Model file for the job. Use its own axes, mm. A direction names the side the tool comes from. Round coordinates to 2 decimals unless told otherwise and drop trailing zeros. Loops run counter-clockwise (first coordinate to the right, second up) from the corner with the lowest first, then second, coordinate; pieces in that order, holes last. Notation, with made-up numbers: M 53.5,75.5 L 68.5,75.5 A15 cw 68.5,94.5 Z; hole C 66,-4 d7. An arc over 180 degrees is marked long. Use a Markdown table: item, result. Add a question column.
Item 1: Pin check, flat tips, straight feed: P1, Ø1, axis at x = -95, z = 9, coming from the +Y side; P2, Ø1.5, axis at x = -96, y = 41.5, coming from the +Z side; P3, Ø2, axis at y = 33, z = 11.5, coming from the +X side; P4, Ø2.5, axis at x = -86, y = 40, coming from the +Z side. Stop position of each tip, or through.
Item 2: Tool access for faces 1 (the flat face through (-96.18, 33.99, 11.52)), 2 (the flat face through (-84.7, 38.7, 13)): list every direction of +Z, -Z, +X, -X, +Y, -Y with a clear straight run to the whole face (end or side of a thin tool).
Item 3: Saw through at C-C on x = -93. Write the cut outline in (y, z).
Item 4: Wall check: L1, parallel to X at y = 40, z = 9.45; L2, parallel to X at y = 40, z = 10.7; L3, parallel to Y at x = -93, z = 9.45. Give the ranges that are in metal, low to high. Write a range as from..to.
Item 5: Two-plate mould, pull along X, no slides. Class faces 3 (the flat face through (-89.82, 46.01, 11.52)), 4 (the flat face through (-93, 43, 8)), 5 (the cylindrical face through (-89.99, 49.536, 10.465)): +X half, -X half, draft (parallel to the pull), parting line (faces both ways), or undercut.
Item 6: Saw through at A-A on y = 40. Write the cut outline in (x, z).
Item 7: Saw through at B-B on z = 10.8. Write the cut outline in (x, y).
Item 8: Saw through at D-D on x = -99.5. Write the cut outline in (y, z), then the cut area to 3 significant figures.
```python
from build123d import *

# Parameters (mm, degrees)
SKETCH042_R             = 10
PAD013_DEPTH            = 5
POCKET026_DEPTH         = 3
SKETCH044_R             = 2.75
POCKET027_DEPTH         = 5.001
SKETCH045_R             = 1.6
POCKET028_DEPTH         = 5.001
BODY008_PLACEMENT_ANGLE = 135


with BuildPart() as part:
    # Sketch042 → Pad013 (new body)
    with BuildSketch(Plane.XY):
        Circle(SKETCH042_R)
    extrude(amount=PAD013_DEPTH)

    # Sketch043 (on Face3 of Pad013) → Pocket026 (cut)
    with BuildSketch(Plane.XY.offset(5)):
        with BuildLine():
            Line((-2, 10), (2, 10))
            Line((2, 10), (2, 3.3))
            ThreePointArc((2, 3.3), (2.380761, 2.380761), (3.3, 2))
            Line((3.3, 2), (10, 2))
            Line((10, 2), (10, -2))
            Line((10, -2), (3.3, -2))
            ThreePointArc((3.3, -2), (2.380761, -2.380761), (2, -3.3))
            Line((2, -3.3), (2, -10))
            Line((2, -10), (-2, -10))
            Line((-2, -10), (-2, -3.3))
            ThreePointArc((-2, -3.3), (-2.380761, -2.380761), (-3.3, -2))
            Line((-3.3, -2), (-10, -2))
            Line((-10, -2), (-10, 2))
            Line((-10, 2), (-3.3, 2))
            ThreePointArc((-3.3, 2), (-2.380761, 2.380761), (-2, 3.3))
            Line((-2, 3.3), (-2, 10))
        make_face()
    extrude(amount=-POCKET026_DEPTH, mode=Mode.SUBTRACT)

    # Sketch044 (on Face2 of Pocket026) → Pocket027 (cut, through all)
    with BuildSketch(Plane(origin=(0, 0, 0), x_dir=(1, 0, 0), z_dir=(0, 0, -1))):
        Circle(SKETCH044_R)
    extrude(amount=-POCKET027_DEPTH, mode=Mode.SUBTRACT)

    # Sketch045 (on Face8 of Pocket027) → Pocket028 (cut, through all)
    with BuildSketch(Plane.XY.offset(5)):
        with Locations((4.949747, 4.949747)):
            Circle(SKETCH045_R)
        with Locations((-4.949747, -4.949747)):
            Circle(SKETCH045_R)
    extrude(amount=-POCKET028_DEPTH, mode=Mode.SUBTRACT)


with BuildPart() as part_1:
    # Body008 placement: moved
    add(part.part.moved(Location((-93, 40, 8))).rotate(Axis((-93, 40, 8), (0, 0, 1)), BODY008_PLACEMENT_ANGLE))


solid = part_1.part
```
Entries:
| question | item | result |
|---|---|---|
| 1 | P1 | y = 49.89 |
| 1 | P2 | z = 10 |
| 1 | P3 | x = -87.83 |
| 1 | P4 | through |
| 2 | face 1 | +Z |
| 2 | face 2 | +Z, +X, -X, +Y, -Y |
| 3 | outline | M 30,8 L 37.25,8 L 37.25,10 L 36.63,10 L 36.63,13 L 30,13 Z; M 42.75,8 L 50,8 L 50,13 L 43.37,13 L 43.37,10 L 42.75,10 Z |
| 4 | L1 | -103..-101.6, -98.4..-95.75, -90.25..-87.6, -84.4..-83 |
| 4 | L2 | -103..-101.6, -98.4..-96.37, -89.63..-87.6, -84.4..-83 |
| 4 | L3 | 30..37.25, 42.75..50 |
| 5 | face 3 | undercut |
| 5 | face 4 | draft |
| 5 | face 5 | parting line |
| 6 | outline | M -103,8 L -101.6,8 L -101.6,13 L -103,13 Z; M -98.4,8 L -95.75,8 L -95.75,10 L -96.37,10 L -96.37,13 L -98.4,13 Z; M -90.25,8 L -87.6,8 L -87.6,13 L -89.63,13 L -89.63,10 L -90.25,10 Z; M -84.4,8 L -83,8 L -83,13 L -84.4,13 Z |
| 7 | outline | M -101.34,34.49 L -96.75,39.08 A1.3 ccw -96.75,40.92 L -101.34,45.51 A10 ccw Z; M -98.51,31.66 A10 ccw -87.49,31.66 L -92.08,36.25 A1.3 ccw -93.92,36.25 Z; M -98.51,48.34 L -93.92,43.75 A1.3 ccw -92.08,43.75 L -87.49,48.34 A10 ccw Z; M -89.25,39.08 L -84.66,34.49 A10 ccw -84.66,45.51 L -89.25,40.92 A1.3 ccw Z; hole C -100,40 d3.2; hole C -86,40 d3.2 |
| 8 | outline | M 32.4,8 L 38.48,8 L 38.48,13 L 36.33,13 L 36.33,10 L 32.4,10 Z; M 41.52,8 L 47.6,8 L 47.6,10 L 43.67,10 L 43.67,13 L 41.52,13 Z |
| 8 | area | 37.2 mm2 |
